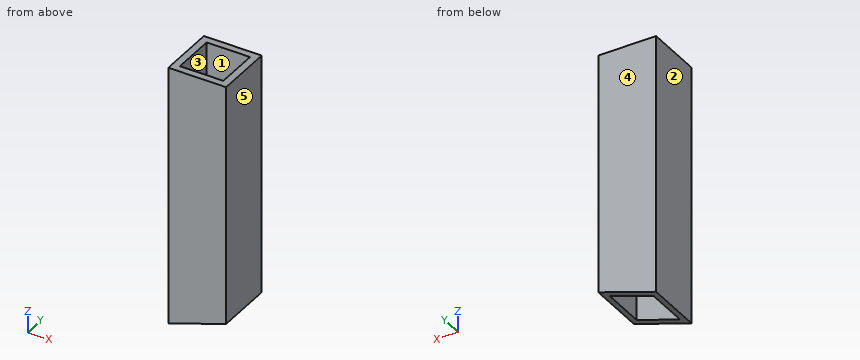
from build123d import *

# Parameters (mm, degrees)
SKETCH1_W           = 25.4
SKETCH1_H           = 25.4
SKETCH1_W_2         = 19.05
SKETCH1_H_2         = 19.05
BOSS_EXTRUDE1_DEPTH = 114.3
CUT_EXTRUDE1_DEPTH  = 120.811560377


with BuildPart() as part:
    # Sketch1 → Boss-Extrude1 (new body)
    with BuildSketch(Plane.XY):
        with Locations((12.7, 12.7)):
            Rectangle(SKETCH1_W, SKETCH1_H)
        with Locations((12.7, 12.7)):
            Rectangle(SKETCH1_W_2, SKETCH1_H_2, mode=Mode.SUBTRACT)
    extrude(amount=BOSS_EXTRUDE1_DEPTH)

    # Sketch2 → Cut-Extrude1 (cut, through all)
    with BuildSketch(Plane(origin=(0, 25.4, 0), x_dir=(1, 0, 0), z_dir=(0, 1, 0))):
        Polygon((0, 0), (25.4, -8.469154802), (25.4, 0), align=None)
    extrude(amount=-CUT_EXTRUDE1_DEPTH, mode=Mode.SUBTRACT)


solid = part.part
For this review, take the finished solid that the model builds, in its own axes (mm). Face numbers are marked on the shaded views. A direction names the side the tool comes from. Round coordinates to 2 decimals unless told otherwise and drop trailing zeros. Write each loop counter-clockwise with the first axis right and the second up, starting at its lowest first coordinate (ties: lowest second). Pieces come first, ordered by that corner, then holes. Notation, with made-up numbers: (60, 38.25) -> (75, 38.25) arc R13 cw to (75, 56.25) -> close; hole circle Ø5 at (-26, 77). An arc over 180 degrees is marked (long way). Use CSV: the item, a comma, the result in double quotes.
(1) Consider section C-C, the plane x = 15. Give the boundary of the cut face in (y, z) (3 decimals).
Computed values:
outline,"(0, 5.001) -> (3.175, 5.001) -> (3.175, 114.3) -> (0, 114.3) -> close; (22.225, 5.001) -> (25.4, 5.001) -> (25.4, 114.3) -> (22.225, 114.3) -> close"
(2) Consider section A-A, the plane y = 6.5. Give the boundary of the cut face in (x, z) (3 decimals), plus the area to 3 significant figures.
Computed values:
outline,"(0, 0) -> (3.175, 1.059) -> (3.175, 114.3) -> (0, 114.3) -> close; (22.225, 7.411) -> (25.4, 8.469) -> (25.4, 114.3) -> (22.225, 114.3) -> close"
area,"699 mm²"
(3) Consider section D-D, the plane y = 23.75. Give the boundary of the cut face in (x, z), plus the area to 3 significant figures.
Computed values:
outline,"(0, 0) -> (25.4, 8.47) -> (25.4, 114.3) -> (0, 114.3) -> close"
area,"2,800 mm²"
(4) To check wall thickness, follow L1, parallel to X at y = 5.25, z = 77 (3 decimals); L2, parallel to Z at x = 24.25, y = 18.75. State the ranges of each line that lie inside material, in increasing order. Write a range as [from, to].
Computed values:
L1,"[0, 3.175], [22.225, 25.4]"
L2,"[8.09, 114.3]"
(5) For the marked faces 1 and 2, list the 3-axis set-ups (+Z, -Z, +X, -X, +Y, -Y) from which the entire face can be reached by the end or side of a thin tool; tool diameter is ignored.
Computed values:
face 1,"+Z, -Z"
face 2,"+Z, -Z, -X, +Y, -Y"
(6) Consider section B-B, the plane z = 36. Give the boundary of the cut face in (x, y) (3 decimals).
Computed values:
outline,"(0, 0) -> (25.4, 0) -> (25.4, 25.4) -> (0, 25.4) -> close; hole (3.175, 3.175) -> (22.225, 3.175) -> (22.225, 22.225) -> (3.175, 22.225) -> close"
(7) Draft analysis for pull direction Y (two halves, no side actions). For the marked faces 3, 4 and 5, state which applies: +Y half, -Y half, draft (parallel to the pull), parting line (faces both ways), or undercut.
Computed values:
face 3,"undercut"
face 4,"+Y half"
face 5,"draft"
(8) Clearance check with a flat-ended pin moving along its axis: P1, Ø8, axis at x = 19.5, z = 72.5, coming from the -Y side. State where the tip first meets the part, or that it passes through.
Computed values:
P1,"y = 0"
